Model file for the job. Use its own axes, mm. A direction names the side the tool comes from. Round coordinates to 2 decimals unless told otherwise and drop trailing zeros. Loops run counter-clockwise (first coordinate to the right, second up) from the corner with the lowest first, then second, coordinate; pieces in that order, holes last. Notation, with made-up numbers: (3, 56) -> (10, 56) arc R23 cw to (10, 77) -> close; hole circle Ø11 at (88.5, -3.75). An arc over 180 degrees is marked (long way). Use a Markdown table: item, result.
from build123d import *

# Parameters (mm, degrees)
BOSS_EXTRUDE2_DEPTH = 15
CUT_EXTRUDE2_DEPTH  = 8
SKETCH5_R           = 4
BOSS_EXTRUDE3_DEPTH = 0.5
BOSS_EXTRUDE3_TAPER = 45
SKETCH6_R           = 2.5
CUT_EXTRUDE3_DEPTH  = 2
SKETCH7_R           = 4.5
CUT_EXTRUDE4_DEPTH  = 5.5
CUT_EXTRUDE5_DEPTH  = 15
SKETCH9_R           = 3
CUT_EXTRUDE6_DEPTH  = 3
SKETCH10_R          = 1.6
CUT_EXTRUDE7_DEPTH  = 4


with BuildPart() as part:
    # Sketch1 → Boss-Extrude2 (new body)
    with BuildSketch(Plane(origin=(0, 0, 0), x_dir=(1, 0, 0), z_dir=(0, 1, 0))):
        with BuildLine():
            Line((0, 0), (16, 0))
            Line((16, 0), (23.390481349, 7.390481349))
            ThreePointArc((23.390481349, 7.390481349), (25.353150018, 8.467238253), (27.586989047, 8.320824708))
            Line((27.586989047, 8.320824708), (36.044222635, 5.242643418))
            ThreePointArc((36.044222635, 5.242643418), (41.811930073, 7.932169566), (39.122403924, 13.699877005))
            Line((39.122403924, 13.699877005), (32.638524841, 16.059815994))
            ThreePointArc((32.638524841, 16.059815994), (30.799841796, 17.427631209), (30.013713531, 19.580228745))
            ThreePointArc((30.013713531, 19.580228745), (25.528138256, 24.7554842), (19.368312088, 21.762125528))
            Line((19.368312088, 21.762125528), (13, 6))
            Line((13, 6), (0, 6))
            Line((0, 6), (0, 0))
        make_face()
    extrude(amount=BOSS_EXTRUDE2_DEPTH)

    # Sketch4 → Cut-Extrude2 (cut)
    with BuildSketch(Plane(origin=(0, 15, 0), x_dir=(1, 0, 0), z_dir=(0, 1, 0))):
        with BuildLine():
            Line((27.527056586, 7.82026535), (39.563282013, 1.837894564))
            Line((39.563282013, 1.837894564), (45.039561208, 12.855889478))
            Line((45.039561208, 12.855889478), (34.588386796, 18.050441613))
            ThreePointArc((34.588386796, 18.050441613), (16.380660644, 23.066124632), (27.527056586, 7.82026535))
        make_face()
    extrude(amount=-CUT_EXTRUDE2_DEPTH, mode=Mode.SUBTRACT)

    # Sketch5 → Boss-Extrude3 (add)
    with BuildSketch(Plane(origin=(0, 7, 0), x_dir=(1, 0, 0), z_dir=(0, 1, 0))):
        with Locations((24.610518338, 17.385504743)):
            Circle(SKETCH5_R)
    extrude(amount=BOSS_EXTRUDE3_DEPTH, taper=BOSS_EXTRUDE3_TAPER)

    # Sketch6 → Cut-Extrude3 (cut)
    with BuildSketch(Plane(origin=(0, 7.5, 0), x_dir=(1, 0, 0), z_dir=(0, 1, 0))):
        with Locations((24.610518338, 17.385504743)):
            Circle(SKETCH6_R)
    extrude(amount=-CUT_EXTRUDE3_DEPTH, mode=Mode.SUBTRACT)

    # Sketch7 → Cut-Extrude4 (cut)
    with BuildSketch(Plane.XZ):
        with Locations((24.610518338, -17.385504743)):
            Circle(SKETCH7_R)
    extrude(amount=-CUT_EXTRUDE4_DEPTH, mode=Mode.SUBTRACT)

    # Sketch8 → Cut-Extrude5 (cut)
    with BuildSketch(Plane.XY):
        with BuildLine():
            Line((4.3, 11.307669683), (4.3, 15))
            Line((4.3, 15), (9.7, 15))
            Line((9.7, 15), (9.7, 11.307669683))
            ThreePointArc((9.7, 11.307669683), (7, 7), (4.3, 11.307669683))
        make_face()
    extrude(amount=-CUT_EXTRUDE5_DEPTH, mode=Mode.SUBTRACT)

    # Sketch9 → Cut-Extrude6 (cut)
    with BuildSketch(Plane(origin=(0, 7, 0), x_dir=(1, 0, 0), z_dir=(0, 1, 0))):
        with Locations((37.583313279, 9.471260211)):
            Circle(SKETCH9_R)
    extrude(amount=-CUT_EXTRUDE6_DEPTH, mode=Mode.SUBTRACT)

    # Sketch10 → Cut-Extrude7 (cut)
    with BuildSketch(Plane(origin=(0, 4, 0), x_dir=(1, 0, 0), z_dir=(0, 1, 0))):
        with Locations((37.583313279, 9.471260211)):
            Circle(SKETCH10_R)
    extrude(amount=-CUT_EXTRUDE7_DEPTH, mode=Mode.SUBTRACT)


solid = part.part
Q1. Tool access for faces 5 (the face through (31.76, 3.45, -6.8)), 6 (the face through (26.687, 2.712, -21.378)), 7 (the face through (39, 4, -8)): list every direction of +Z, -Z, +X, -X, +Y, -Y with a clear straight run to the whole face (end or side of a thin tool).
Results list:
| item | result |
|---|---|
| face 5 | +Z, +Y, -Y |
| face 6 | -Y |
| face 7 | +Y |
Q2. Band-saw the part on A-A, the plane y = 12. Give the cut face in (x, z).
Results list:
| item | result |
|---|---|
| outline | (0, -6) -> (4.3, -6) -> (4.3, 0) -> (0, 0) -> close; (9.7, -6) -> (13, -6) -> (15.74, -12.77) arc R10 cw to (23.45, -7.45) arc R4 cw to (23.39, -7.39) -> (16, 0) -> (9.7, 0) -> close |
Q3. Band-saw the part on B-B, the plane y = 1.5. Give the number of separate pieces and of enclosed holes in the cut face, plus the area to 3 significant figures.
Results list:
| item | result |
|---|---|
| separate pieces | 1 |
| enclosed holes | 2 |
| area | 373 mm² |
Q4. Drill centre lines: L1, parallel to Z at x = 25, y = 6.5; L2, parallel to X at y = 2.25, z = -20.75; L3, parallel to Z at x = 3, y = 8.25. Where is each one in solid material? Low to high. Write a range as from..to.
Results list:
| item | result |
|---|---|
| L1 | z = -24.84..-19.85, -14.92..-8.37 |
| L2 | x = 18.96..21.62, 27.6..29.82 |
| L3 | z = -6..0 |
Q5. Band-saw the part on D-D, the plane x = 35. Give the cut face in (y, z), plus the area to 3 significant figures.
Results list:
| item | result |
|---|---|
| outline | (0, -15.2) -> (7, -15.2) -> (7, -11) -> (4, -11) -> (4, -7.95) -> (7, -7.95) -> (7, -5.62) -> (0, -5.62) -> close |
| area | 57.9 mm² |
Q6. Pull direction X, two halves, no side cores. Call faces 1 (the face through (30.82, 3.45, -17.4)), 2 (the face through (35.985, 2.028, -9.542)), 3 (the face through (0, 7, -3)), 4 (the face through (7, 6, -6)): released by +X, released by -X, zero draft, split by the parting line, or undercut.
Results list:
| item | result |
|---|---|
| face 1 | released by +X |
| face 2 | undercut |
| face 3 | released by -X |
| face 4 | zero draft |
Q7. Flat gauge pins, fed straight in: pin 1 (10 mm diameter, centred on x = 23, z = -3, fed in from +Y); pin 2 (2.5 mm diameter, centred on x = 25, z = -15.5, fed in from -Y); pin 3 (11.5 mm diameter, centred on x = 24.61, z = -17.39, fed in from +Y); pin 4 (6.5 mm diameter, centred on x = 5, y = 6, fed in from -Z). Where does each tip first touch, or does it go through?
Results list:
| item | result |
|---|---|
| pin 1 | stops at y = 15 |
| pin 2 | stops at y = 5.5 |
| pin 3 | stops at y = 7.5 |
| pin 4 | stops at z = -6 |
Q8. Band-saw the part on C-C, the plane z = -4.25. Give the cut face in (x, y), plus the area to 3 significant figures.
Results list:
| item | result |
|---|---|
| outline | (0, 0) -> (20.25, 0) -> (20.25, 15) -> (9.7, 15) -> (9.7, 11.31) arc R3 cw (long way) to (4.3, 11.31) -> (4.3, 15) -> (0, 15) -> close |
| area | 262 mm² |
